The listing builds one solid part. Answer for the finished solid, in the listing's coordinates (mm). A direction names the side the tool comes from. Give positions to 0.01 mm unless a question says otherwise; leave off trailing zeros. Write each loop counter-clockwise with the first axis right and the second up, starting at its lowest first coordinate (ties: lowest second). Pieces come first, ordered by that corner, then holes. Notation, with made-up numbers: (76.25, -14) - (121.25, -14) arc R24 cw to (121.25, 4) - close; hole circle Ø11 at (-14, 36.25). An arc over 180 degrees is marked (long way). One line per item, written item: value. Start each with the question number.
Autodesk Inventor part; units mm, degrees
ref_plane "YZ Plane" through (0, 0, 0) normal (1, 0, 0) x (0, 1, 0)
ref_plane "XZ Plane" through (0, 0, 0) normal (0, 1, 0) x (-1, 0, 0)
ref_plane "XY Plane" through (0, 0, 0) normal (0, 0, 1) x (1, 0, 0)
sketch "Sketch1" plane through (0, 0, 0) normal (0, 1, 0) x (-1, 0, 0)
  line L0 (-13.5, -18.4952) -> (9.75, -18.4952)
  line L1 (9.75, -18.4952) -> (9.75, 18.4952)
  line L2 (9.75, 18.4952) -> (-13.5, 18.4952)
  line L3 (-13.5, 18.4952) -> (-13.5, -18.4952)
  circle A0 centre (-7.5, 0) radius 4
  circle A1 centre (3.75, -6.4952) radius 4
  circle A2 centre (3.75, 6.4952) radius 4
  circle A3 centre (0, 0) radius 7.5 construction
  circle A4 centre (0, 0) radius 2.5
  dimension "d11" = 15
  dimension "d2" = 8
  dimension "d6" = 360
  dimension "d8" = 6
  dimension "d9" = 6
  dimension "d1" = 12
  dimension "d13" = 12
  dimension "d35" = 5
extrude "Extrusion1" add sketch "Sketch1" along normal blind 4
sketch "Sketch2" plane through (0, 4, 0) normal (0, 1, 0) x (1, 0, 0)
  circle A0 centre (-3.75, -6.4952) radius 4
  circle A1 centre (-3.75, 6.4952) radius 4
  circle A2 centre (7.5, 0) radius 4
  line L0 (13.5, 18.4952) -> (-9.75, 18.4952)
  line L1 (-9.75, 18.4952) -> (-9.75, -18.4952)
  line L2 (-9.75, -18.4952) -> (13.5, -18.4952)
  line L3 (13.5, -18.4952) -> (13.5, 18.4952)
  circle A3 centre (0, 0) radius 2.5
  dimension "d16" = 5
extrude "Extrusion2" add sketch "Sketch2" along normal blind 1 contours A0 | A1 | A2 | L3 L2 L1 L0
sketch "Sketch3" plane through (0, 0, 0) normal (0, -1, 0) x (1, 0, 0)
  circle A0 centre (-3.75, 6.4952) radius 4
  circle A1 centre (-3.75, -6.4952) radius 4
  circle A2 centre (7.5, 0) radius 4
  line L0 (13.5, -18.4952) -> (-9.75, -18.4952)
  line L1 (13.5, 18.4952) -> (13.5, -18.4952)
  line L2 (-9.75, 18.4952) -> (13.5, 18.4952)
  line L3 (-9.75, -18.4952) -> (-9.75, 18.4952) construction
  line L4 (-1.5, 18.4952) -> (13.5, 9.4952)
  line L5 (13.5, 18.4952) -> (13.5, -18.4952)
  line L6 (13.5, -9.4952) -> (-1.5, -18.4952)
  point P0 (0, 0)
  dimension "d19" = 9
  dimension "d20" = 9
  dimension "d21" = 15
  dimension "d22" = 15
extrude "Extrusion3" cut sketch "Sketch3" against normal through all contours L4 L2 L1 | L0 L6 L1
sketch "Sketch5" plane through (0, 0, 0) normal (0, -1, 0) x (1, 0, 0)
  line L0 (13.5, 9.4952) -> (-1.5, 18.4952)
  line L1 (-9.75, 18.4952) -> (-1.5, 18.4952)
  line L2 (-9.75, -18.4952) -> (-9.75, 18.4952)
  line L3 (-1.5, -18.4952) -> (-9.75, -18.4952)
  line L4 (-1.5, -18.4952) -> (13.5, -9.4952)
  line L5 (13.5, 9.4952) -> (13.5, -9.4952)
  circle A0 centre (-3.75, 6.4952) radius 4
  circle A1 centre (-3.75, -6.4952) radius 4
  circle A2 centre (7.5, 0) radius 4
  line L6 (17.5, -11.76) -> (-0.3921, -22.4952)
  line L7 (-0.3921, -22.4952) -> (-13.75, -22.4952)
  line L8 (-13.75, -22.4952) -> (-13.75, 22.4952)
  line L9 (-13.75, 22.4952) -> (-0.3921, 22.4952)
  line L10 (-0.3921, 22.4952) -> (17.5, 11.76)
  line L11 (17.5, 11.76) -> (17.5, -11.76)
  line L12 (13.5, -9.4952) -> (13.5, -14.16)
  line L13 (13.5, 3.4118) -> (13.5, 14.16)
  line L14 (-1.5, -18.4952) -> (-9.75, -18.4952)
  line L15 (-9.75, -18.4952) -> (-9.75, -22.4952)
  line L16 (-9.75, 18.4952) -> (-1.5, 18.4952)
  line L17 (-9.75, 18.4952) -> (-9.75, 22.4952)
  line L18 (-1.5, -18.4952) -> (13.5, -9.4952)
  line L19 (13.5, -9.4952) -> (-1.5, -18.4952)
  line L20 (-1.5, -18.4952) -> (-9.75, -18.4952)
  line L21 (-9.75, -18.4952) -> (-9.75, 18.4952)
  line L22 (-9.75, 18.4952) -> (-1.5, 18.4952)
  line L23 (13.5, 9.4952) -> (-1.5, 18.4952)
  line L24 (13.5, 9.4952) -> (-1.5, 18.4952)
  line L25 (13.5, -9.4952) -> (13.5, 3.4118)
  point P0 (0, 0)
  dimension "d27" = 4
extrude "Extrusion5" add sketch "Sketch5" against normal up to surface (5 mm away) contours L0 L1 L17 L9 L10 L13 | L12 L6 L7 L15 L3 L4
sketch "Sketch6" plane through (0, 5, 0) normal (0, 1, 0) x (1, 0, 0)
  line L0 (13.5, -14.16) -> (13.5, 14.16)
  line L1 (-0.3921, 22.4952) -> (13.5, 14.16)
  line L2 (-9.75, 22.4952) -> (-0.3921, 22.4952)
  line L3 (-9.75, -22.4952) -> (-9.75, 22.4952)
  line L4 (-0.3921, -22.4952) -> (-9.75, -22.4952)
  line L5 (13.5, -14.16) -> (-0.3921, -22.4952)
  line L6 (13.5, 14.16) -> (-0.3921, 22.4952)
  line L7 (-0.3921, 22.4952) -> (-1.9356, 19.9227)
  line L8 (-1.9356, 19.9227) -> (11.9565, 11.5875)
  line L9 (11.9565, 11.5875) -> (13.5, 14.16)
  line L10 (13.5, -14.16) -> (13.5, 14.16)
  line L11 (13.5, -14.16) -> (-0.3921, -22.4952)
  line L12 (-0.3921, -22.4952) -> (-1.9356, -19.9227)
  line L13 (-1.9356, -19.9227) -> (11.9565, -11.5875)
  line L14 (11.9565, -11.5875) -> (13.5, -14.16)
  point P0 (0, 0)
  dimension "d30" = 3
  dimension "d31" = 3
extrude "Extrusion6" add sketch "Sketch6" along normal blind 10 contours L5 L12 L13 L14 | L9 L8 L7 L1
chamfer "Chamfer1" distance 0.5 angle 45 5 edges at (2.5, 0, 0) (-2.5, 5, 0) (0.25, 0, 6.4952) (11.5, 0, 0) (0.25, 0, -6.4952)
equation "\"d13\" = d1"
properties part number "30_Cube_Z_Focus_Drylin_NEMA_slide_part1"
Item 1: The mould has two halves that part along X. Classify faces 6 (the flat face through (13.5, 2, 0)), 7 (the flat face through (-1.15, 9.93, 21.23)), 8 (the flat face through (7, 4, 0)): +X half, -X half, draft (parallel to the pull), parting line (faces both ways), or undercut.
Item 2: Straight lines are drawn through the part: line 1 along Z through (x, y) = (-3.75, 2.35); line 2 along Y through (x, z) = (-6, -1.5); line 3 along Y through (x, z) = (-6.25, -4). For each, find the intervals that lie inside material, in ascending order.
Item 3: Find section C-C on z = -17.5. Determine the outline of the cut face in (x, y).
Item 4: Find section A-A on y = 11.5. Determine the outline of the cut face in (x, z).
Item 5: Find section B-B on x = -3.75. Determine the outline of the cut face in (y, z), plus the area to 3 significant figures.
Item 6: Find section D-D on z = 13. Determine the outline of the cut face in (x, y).
Item 7: Each of these flat-tipped pins is pushed along its axis until it touches: pin 1 Ø1.5 at (x, y) = (9.5, 12.5) entering from +Z; pin 2 Ø6 at (x, z) = (4.5, 7) entering from -Y; pin 3 Ø1.5 at (y, z) = (9.5, 11.5) entering from +X; pin 4 Ø2.5 at (x, z) = (-4, -7) entering from -Y. Where does it stop, or does it pass through?
Item 8: For faces 1 (the flat face through (-4, 4, -7)), 2 (the flat face through (-1.15, 9.93, -21.23)), 3 (the flat face through (12.72, 9.93, 12.86)), 4 (the flat face through (4.913, 9.93, 15.813)), 5 (the flat face through (6, 15, -17)), determine the directions among +Z, -Z, +X, -X, +Y, -Y from which every point of the face is accessible in a straight line to the end or side of a thin tool.
Values:
1. face 6: +X half
1. face 7: -X half
1. face 8: undercut
2. line 1: -22.5 to -10.5, -2.5 to 2.5, 10.5 to 22.5
2. line 2: 0 to 5
2. line 3: 4 to 5
3. outline: (-9.75, 0) - (7.93, 0) - (7.93, 15) - (2.1, 15) - (2.1, 5) - (-9.75, 5) - close
4. outline: (-1.94, -19.92) - (-0.39, -22.5) - (13.5, -14.16) - (11.96, -11.59) - close; (-1.94, 19.92) - (11.96, 11.59) - (13.5, 14.16) - (-0.39, 22.5) - close
5. outline: (0, -22.5) - (5, -22.5) - (5, 22.5) - (0, 22.5) - (0, 10.99) - (0.5, 10.5) - (4, 10.5) - (4, 2.5) - (0.5, 2.5) - (0, 2) - (0, -2) - (0.5, -2.5) - (4, -2.5) - (4, -10.5) - (0.5, -10.5) - (0, -10.99) - close
5. area: 160 mm^2
6. outline: (-9.75, 0) - (13.5, 0) - (13.5, 5) - (12.8, 5) - (12.8, 15) - (9.6, 15) - (9.6, 5) - (-9.75, 5) - close
7. pin 1: z = 17.01
7. pin 2: y = 0
7. pin 3: x = 12.35
7. pin 4: y = 4
8. face 1: -Y
8. face 2: -Z, -X, +Y
8. face 3: +X, +Y
8. face 4: -X, +Y
8. face 5: +Z, -Z, +X, -X, +Y
